Here's how the part is built. I have some questions about the finished solid (model axes, mm). Coordinates: 2 decimals unless noted, no trailing zeros. Order: outer loops, then holes, each group sorted by start corner. A loop starts at its lowest first (then second) coordinate and runs counter-clockwise, first axis right, second up. Notation, with made-up numbers: (-27.75, -37.75) - (1.25, -37.75) arc R26 cw to (1.25, -17.75) - close; hole circle Ø10 at (45, 86.25). An arc over 180 degrees is marked (long way). Use one line per item in the form item = value. Start each with the question number.
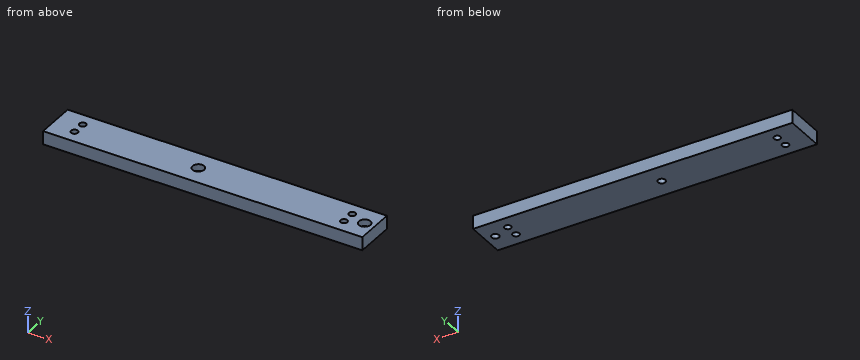
from build123d import *

# Parameters (mm, degrees)
F0_W           = 609.6
F0_H           = 76.2
F1_DEPTH       = 25.4
F2_R           = 6.35
F3_DEPTH       = 25.4
F5_D           = 14.2875
F5_CBORE_D     = 22.225
F5_CBORE_DEPTH = 12.7


with BuildPart() as f1:
    # F0 (on Top) → F1 (new body)
    with BuildSketch(Plane.XY):
        Rectangle(F0_W, F0_H)
    extrude(amount=F1_DEPTH)

    # F2 (on face) → F3 (cut)
    with BuildSketch(Plane.XY.offset(25.4)):
        with Locations((254, -12.7)):
            Circle(F2_R)
        with Locations((254, 12.7)):
            Circle(F2_R)
        with Locations((-260.35, -12.7)):
            Circle(F2_R)
        with Locations((-260.35, 12.7)):
            Circle(F2_R)
    extrude(amount=-F3_DEPTH, mode=Mode.SUBTRACT)

    # F5 (through all)
    with Locations(Plane.XY.offset(25.4)):
        with Locations((-31.75, 0), (285.75, 0)):
            CounterBoreHole(F5_D / 2, F5_CBORE_D / 2, F5_CBORE_DEPTH)


solid = f1.part
1) I need wall thicknesses on probe 1 along Y at (x, z) = (-260.35, 10); probe 2 along Y at (x, z) = (-263, 11.25); probe 3 along X at (y, z) = (-16, 3). Which ranges of each line are inside material? Lowest first, please. Write a range as [from, to].
2) Suppose I cut it at B-B, the plane x = 254. List the corners of the cut face in (y, z) for me.
3) Suppose I cut it at C-C, the plane z = 20. Give the number of separate pieces and of enclosed holes in the cut face, then the cut area to 3 significant figures.
4) Suppose I cut it at D-D, the plane x = -31.75. List the corners of the cut face in (y, z) for me, then the cut area to 3 significant figures.
5) For pin 1 (13.5 mm diameter, centred on x = 285.75, y = 0, fed in from +Z); pin 2 (11 mm diameter, centred on x = -35.5, y = 2.5, fed in from +Z), each with a flat end and sliding along its axis, tell me the tip position at first contact or that it passes through.
6) Suppose I cut it at A-A, the plane y = 0. List the corners of the cut face in (x, z) for me, then the cut area to 3 significant figures.
From the geometry:
q1.probe_1 = [-38.1, -19.05], [-6.35, 6.35], [19.05, 38.1]
q1.probe_2 = [-38.1, -18.47], [-6.93, 6.93], [18.47, 38.1]
q1.probe_3 = [-304.8, -265.78], [-254.92, 248.57], [259.43, 304.8]
q2.outline = (-38.1, 0) - (-19.05, 0) - (-19.05, 25.4) - (-38.1, 25.4) - close; (-6.35, 0) - (6.35, 0) - (6.35, 25.4) - (-6.35, 25.4) - close; (19.05, 0) - (38.1, 0) - (38.1, 25.4) - (19.05, 25.4) - close
q3.separate_pieces = 1
q3.enclosed_holes = 6
q3.area = 45,200 mm2
q4.outline = (-38.1, 0) - (-7.14, 0) - (-7.14, 12.7) - (-11.11, 12.7) - (-11.11, 25.4) - (-38.1, 25.4) - close; (7.14, 0) - (38.1, 0) - (38.1, 25.4) - (11.11, 25.4) - (11.11, 12.7) - (7.14, 12.7) - close
q4.area = 1,470 mm2
q5.pin_1 = through
q5.pin_2 = 12.7
q6.outline = (-304.8, 0) - (-38.89, 0) - (-38.89, 12.7) - (-42.86, 12.7) - (-42.86, 25.4) - (-304.8, 25.4) - close; (-24.61, 0) - (278.61, 0) - (278.61, 12.7) - (274.64, 12.7) - (274.64, 25.4) - (-20.64, 25.4) - (-20.64, 12.7) - (-24.61, 12.7) - close; (292.89, 0) - (304.8, 0) - (304.8, 25.4) - (296.86, 25.4) - (296.86, 12.7) - (292.89, 12.7) - close
q6.area = 14,600 mm2
